```python
from build123d import *

# Parameters (mm, degrees)
SKETCH_1_R      = 1.55
SKETCH_1_R_2    = 1.593407699
SKETCH_1_R_3    = 1.506592301
SKETCH_1_R_4    = 1.546583653
SKETCH_1_R_5    = 2
EXTRUDE_1_DEPTH = 4


with BuildPart() as part:
    # 草图1 → 凸台-拉伸1 (new body)
    with BuildSketch(Plane.XY):
        with BuildLine():
            Line((-49.086064172, -18.127823684), (-41.682309555, -18.127823684))
            Line((-41.682309555, -18.127823684), (-17.432309555, -18.127823684))
            ThreePointArc((-17.432309555, -18.127823684), (-10.361241743, -21.056755872), (-7.432309555, -28.127823684))
            Line((-7.432309555, -28.127823684), (-7.432309555, -56.439146577))
            Line((-7.432309555, -56.439146577), (24.519698232, -56.439146577))
            Line((24.519698232, -56.439146577), (24.519698232, -28.127823684))
            ThreePointArc((24.519698232, -28.127823684), (27.44863042, -21.056755872), (34.519698232, -18.127823684))
            Line((34.519698232, -18.127823684), (58.769698232, -18.127823684))
            Line((58.769698232, -18.127823684), (66.173452848, -18.127823684))
            ThreePointArc((66.173452848, -18.127823684), (73.24452066, -15.198891495), (76.173452848, -8.127823684))
            Line((76.173452848, -8.127823684), (27.509504294, 47.847762189))
            ThreePointArc((27.509504294, 47.847762189), (24.109445562, 50.386499783), (19.962749895, 51.28677918))
            Line((19.962749895, 51.28677918), (8.543694338, 51.28677918))
            Line((8.543694338, 51.28677918), (-2.875361218, 51.28677918))
            ThreePointArc((-2.875361218, 51.28677918), (-7.022056885, 50.386499783), (-10.422115617, 47.847762189))
            Line((-10.422115617, 47.847762189), (-59.086064172, -8.127823684))
            ThreePointArc((-59.086064172, -8.127823684), (-56.157131983, -15.198891495), (-49.086064172, -18.127823684))
        make_face()
        with Locations((-1.956305662, -35.174209618)):
            Circle(SKETCH_1_R, mode=Mode.SUBTRACT)
        with Locations((-40.456305662, -8.174209618)):
            Circle(SKETCH_1_R, mode=Mode.SUBTRACT)
        with Locations((-21.414481972, -14.185828882)):
            Circle(SKETCH_1_R_2, mode=Mode.SUBTRACT)
        with Locations((-11.456305662, -14.174209618)):
            Circle(SKETCH_1_R, mode=Mode.SUBTRACT)
        with Locations((-16.414481972, -3.685828882)):
            Circle(SKETCH_1_R_3, mode=Mode.SUBTRACT)
        with Locations((-1.956305662, -14.174209618)):
            Circle(SKETCH_1_R, mode=Mode.SUBTRACT)
        with Locations((8.543694338, -45.674209618)):
            Circle(SKETCH_1_R, mode=Mode.SUBTRACT)
        with Locations((19.043694338, -35.174209618)):
            Circle(SKETCH_1_R, mode=Mode.SUBTRACT)
        with Locations((8.543694338, -24.674209618)):
            Circle(SKETCH_1_R_4, mode=Mode.SUBTRACT)
        with Locations((19.043694338, -14.174209618)):
            Circle(SKETCH_1_R, mode=Mode.SUBTRACT)
        with Locations((8.543694338, -3.674209618)):
            Circle(SKETCH_1_R, mode=Mode.SUBTRACT)
        with Locations((28.543694338, -14.174209618)):
            Circle(SKETCH_1_R, mode=Mode.SUBTRACT)
        with Locations((38.501870648, -14.185828882)):
            Circle(SKETCH_1_R_2, mode=Mode.SUBTRACT)
        with Locations((33.501870648, -3.685828882)):
            Circle(SKETCH_1_R_3, mode=Mode.SUBTRACT)
        with Locations((57.543694338, -8.174209618)):
            Circle(SKETCH_1_R, mode=Mode.SUBTRACT)
        with Locations((-1.956305662, 31.263738804)):
            Circle(SKETCH_1_R_5, mode=Mode.SUBTRACT)
        with Locations((8.543694338, 20.763738804)):
            Circle(SKETCH_1_R_5, mode=Mode.SUBTRACT)
        with Locations((19.043694338, 31.263738804)):
            Circle(SKETCH_1_R_5, mode=Mode.SUBTRACT)
        with Locations((8.543694338, 41.763738804)):
            Circle(SKETCH_1_R_5, mode=Mode.SUBTRACT)
    extrude(amount=EXTRUDE_1_DEPTH)


solid = part.part
```
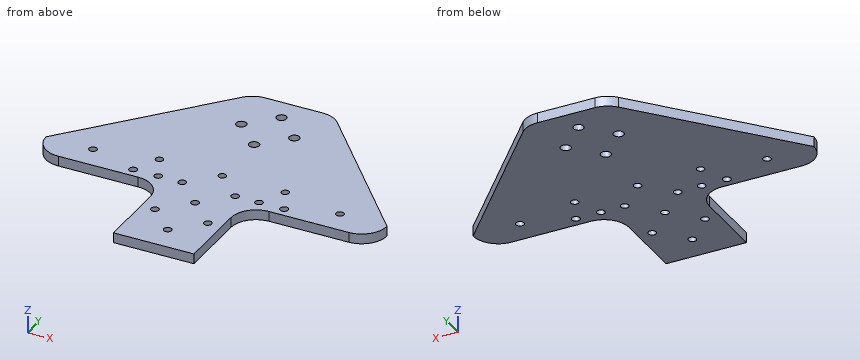
Can you work these out from the model? Positions are in its coordinate system, mm. Coordinates: 2 decimals unless noted, no trailing zeros. Loops run counter-clockwise (first coordinate to the right, second up) from the corner with the lowest first, then second, coordinate; pieces in that order, holes last. Notation, with made-up numbers: (55, 68.5) - (93, 68.5) arc R29 ccw to (93, 104.5) - close; hole circle Ø7 at (-29.5, 78). An arc over 180 degrees is marked (long way). Use a Markdown table: item, result.
Item 1: If I drill on probe 1 along X at (y, z) = (-45.5, 3); probe 2 along X at (y, z) = (33, 3.35); probe 3 along X at (y, z) = (11.5, 1.05), over which ranges is the centre line in solid material (lowest first)? Write a range as from..to.
Numbers:
| item | result |
|---|---|
| probe 1 | x = -7.43..7, 10.08..24.52 |
| probe 2 | x = -23.33..-2.95, -0.96..18.05, 20.04..40.42 |
| probe 3 | x = -42.02..59.11 |
Item 2: I want a section at C-C on y = 13.5. Please give me the cut outline in (x, z).
Numbers:
| item | result |
|---|---|
| outline | (-40.28, 0) - (57.37, 0) - (57.37, 4) - (-40.28, 4) - close |
Item 3: Will these pins go through, and if not, where does the flat tip stop? pin 1 (3.5 mm diameter, centred on x = 19.04, y = -35.17, fed in from +Z); pin 2 (2 mm diameter, centred on y = -40, z = 1.5, fed in from -X).
Numbers:
| item | result |
|---|---|
| pin 1 | stops at z = 4 |
| pin 2 | stops at x = -7.43 |
Item 4: I want a section at B-B on x = -45.5. Please give me the cut outline in (y, z), and give its area (3 significant figures).
Numbers:
| item | result |
|---|---|
| outline | (-18.13, 0) - (7.5, 0) - (7.5, 4) - (-18.13, 4) - close |
| area | 103 mm2 |
Item 5: I want a section at A-A on z = 2.2. Give the number of separate pieces and of enclosed holes in the cut face, and give its area (3 significant figures).
Numbers:
| item | result |
|---|---|
| separate pieces | 1 |
| enclosed holes | 19 |
| area | 7,380 mm2 |
